Here's the drawing with two shaded views (mm, measured from the low corner). I have some questions. A direction names the side the tool comes from. Round coordinates to 2 decimals unless told otherwise and drop trailing zeros. Order: outer loops, then holes, each group sorted by start corner. A loop starts at its lowest first (then second) coordinate and runs counter-clockwise, first axis right, second up. Notation, with made-up numbers: (54.25, 24.5) -> (110.25, 24.5) arc R21 cw to (110.25, 29.5) -> close; hole circle Ø6 at (57, 87). An arc over 180 degrees is marked (long way). Answer in a Markdown table with one row per item.
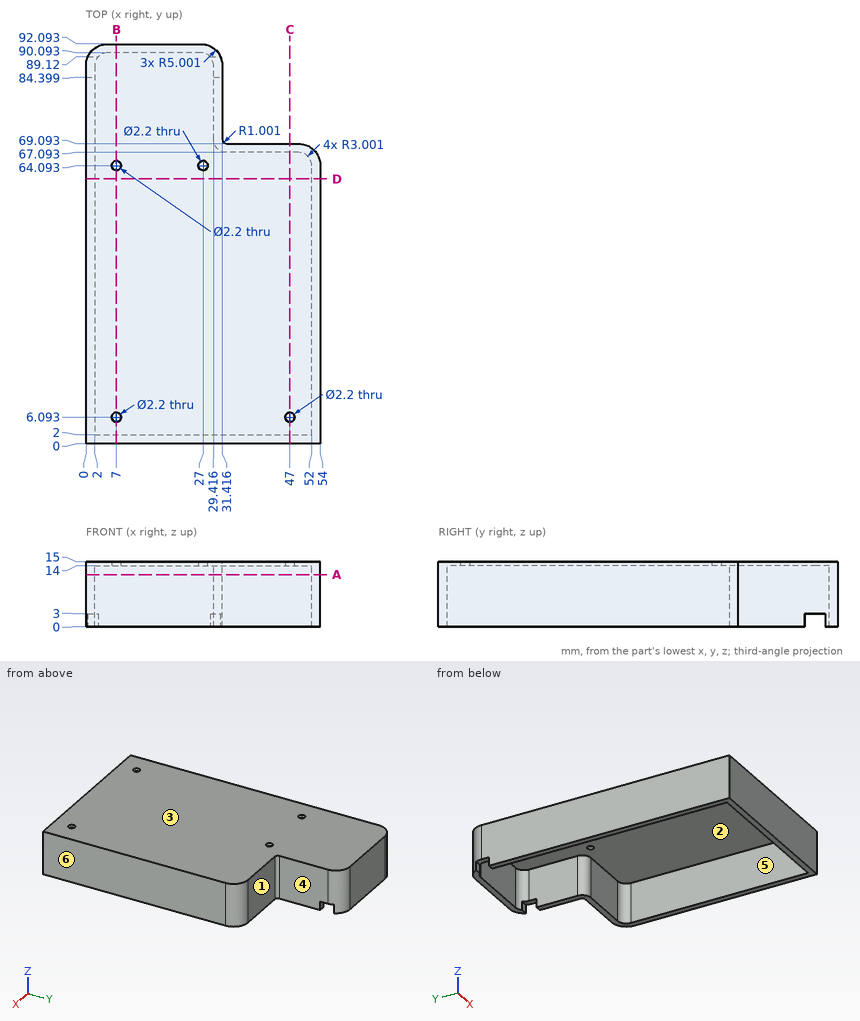
1. Suppose I cut it at B-B on x = 7. Write out the boundary of the cut face in (y, z), then the cut area to 3 significant figures.
Numbers:
| item | result |
|---|---|
| outline | (0, 0) -> (2, 0) -> (2, 14) -> (4.99, 14) -> (4.99, 15) -> (0, 15) -> close; (7.19, 14) -> (62.99, 14) -> (62.99, 15) -> (7.19, 15) -> close; (65.19, 14) -> (90.09, 14) -> (90.09, 0) -> (92.09, 0) -> (92.09, 15) -> (65.19, 15) -> close |
| area | 144 mm2 |
2. Please list where these lines run through material, in increasing order: line 1 along Y through (x, z) = (7.5, 13); line 2 along X through (y, z) = (63, 9.75); line 3 along Y through (x, z) = (47, 14.45).
Numbers:
| item | result |
|---|---|
| line 1 | y = 0 to 2, 90.09 to 92.09 |
| line 2 | x = 0 to 2, 52 to 54 |
| line 3 | y = 0 to 4.99, 7.19 to 69.09 |
3. Suppose I cut it at A-A on z = 12. Write out the boundary of the cut face in (x, y) (1 decimal).
Numbers:
| item | result |
|---|---|
| outline | (0, 0) -> (54, 0) -> (54, 64.1) arc R5 ccw to (49, 69.1) -> (32.4, 69.1) arc R1 cw to (31.4, 70.1) -> (31.4, 87.1) arc R5 ccw to (26.4, 92.1) -> (5, 92.1) arc R5 ccw to (0, 87.1) -> close; hole (2, 2) -> (52, 2) -> (52, 64.1) arc R3 ccw to (49, 67.1) -> (32.4, 67.1) arc R3 cw to (29.4, 70.1) -> (29.4, 87.1) arc R3 ccw to (26.4, 90.1) -> (5, 90.1) arc R3 ccw to (2, 87.1) -> close |
4. For the marked faces 4, 5 and 6, which set-ups out of +Z, -Z, +X, -X, +Y, -Y let a thin tool reach every point of the face, with its end or its side?
Numbers:
| item | result |
|---|---|
| face 4 | +Z, -Z, +X, +Y |
| face 5 | -Z |
| face 6 | +Z, -Z, +X, +Y, -Y |
5. Suppose I cut it at D-D on y = 61. Write out the boundary of the cut face in (x, z).
Numbers:
| item | result |
|---|---|
| outline | (0, 0) -> (2, 0) -> (2, 14) -> (52, 14) -> (52, 0) -> (54, 0) -> (54, 15) -> (0, 15) -> close |
6. Suppose I cut it at C-C on x = 47. Write out the boundary of the cut face in (y, z).
Numbers:
| item | result |
|---|---|
| outline | (0, 0) -> (2, 0) -> (2, 14) -> (4.99, 14) -> (4.99, 15) -> (0, 15) -> close; (7.19, 14) -> (67.09, 14) -> (67.09, 0) -> (69.09, 0) -> (69.09, 15) -> (7.19, 15) -> close |
7. We'd pull the mould along Y, two halves only. Please class the marked faces 1, 2 and 3: released by +Y, released by -Y, zero draft, split by the parting line, or undercut.
Numbers:
| item | result |
|---|---|
| face 1 | released by +Y |
| face 2 | undercut |
| face 3 | zero draft |
8. For pin 1 Ø1.4 at (x, y) = (30, 87) entering from -Z; pin 2 Ø0.6 at (x, z) = (30.5, 2) entering from +Y; pin 3 Ø4 at (y, z) = (69, 2.5) entering from +X; pin 4 Ø2 at (x, y) = (7, 6.09) entering from -Z, each with a flat end and sliding along its axis, tell me the tip position at first contact or that it passes through.
Numbers:
| item | result |
|---|---|
| pin 1 | stops at z = 3 |
| pin 2 | stops at y = 90.36 |
| pin 3 | stops at x = 53.07 |
| pin 4 | passes through |
